from build123d import *

# Parameters (mm, degrees)
SKETCH1_W           = 50
SKETCH1_H           = 110
BOSS_EXTRUDE1_DEPTH = 10
SKETCH2_W           = 12
SKETCH2_H           = 110
BOSS_EXTRUDE2_DEPTH = 120
BOSS_EXTRUDE4_DEPTH = 152
BOSS_EXTRUDE5_DEPTH = 10
SKETCH5_W           = 152
SKETCH5_H           = 8
BOSS_EXTRUDE6_DEPTH = 10
SKETCH6_W           = 152
SKETCH6_H           = 8
BOSS_EXTRUDE7_DEPTH = 10
SKETCH7_R           = 2.5
CUT_EXTRUDE1_DEPTH  = 87
SKETCH8_W           = 26
SKETCH8_H           = 63.5
CUT_EXTRUDE2_DEPTH  = 5


with BuildPart() as part:
    # Sketch1 → Boss-Extrude1 (new body)
    with BuildSketch(Plane.XY):
        with Locations((-25, 55)):
            Rectangle(SKETCH1_W, SKETCH1_H)
    extrude(amount=BOSS_EXTRUDE1_DEPTH)

    # Sketch2 → Boss-Extrude2 (add)
    with BuildSketch(Plane(origin=(0, 0, 0), x_dir=(-1, 0, 0), z_dir=(0, 0, -1))):
        with Locations((6, 55)):
            Rectangle(SKETCH2_W, SKETCH2_H)
    extrude(amount=BOSS_EXTRUDE2_DEPTH)

    # Sketch3 → Boss-Extrude4 (add)
    with BuildSketch(Plane.ZY.offset(12)):
        Polygon((-120, 86.75), (-120, 76.75), (-114, 76.75), (-114, 33.25), (-120, 33.25), (-120, 23.25), (-104, 23.25), (-104, 86.75), align=None)
    extrude(amount=BOSS_EXTRUDE4_DEPTH)

    # Sketch4 → Boss-Extrude5 (add)
    with BuildSketch(Plane(origin=(0, 0, -120), x_dir=(-1, 0, 0), z_dir=(0, 0, -1))):
        Polygon((12, 86.75), (0, 86.75), (0, 23.25), (12, 23.25), (164, 23.25), (164, 33.25), (12, 33.25), (12, 76.75), (164, 76.75), (164, 86.75), align=None)
    extrude(amount=BOSS_EXTRUDE5_DEPTH)

    # Sketch5 → Boss-Extrude6 (add)
    with BuildSketch(Plane.XZ.offset(-76.75)):
        with Locations((-88, -126)):
            Rectangle(SKETCH5_W, SKETCH5_H)
    extrude(amount=BOSS_EXTRUDE6_DEPTH)

    # Sketch6 → Boss-Extrude7 (add)
    with BuildSketch(Plane(origin=(0, 33.25, 0), x_dir=(1, 0, 0), z_dir=(0, 1, 0))):
        with Locations((-88, 126)):
            Rectangle(SKETCH6_W, SKETCH6_H)
    extrude(amount=BOSS_EXTRUDE7_DEPTH)

    # Sketch7 → Cut-Extrude1 (cut)
    with BuildSketch(Plane.XY.offset(-104)):
        with Locations((-124, 61.25)):
            Circle(SKETCH7_R)
        with Locations((-124, 47.25)):
            Circle(SKETCH7_R)
    extrude(amount=-CUT_EXTRUDE1_DEPTH, mode=Mode.SUBTRACT)

    # Sketch8 → Cut-Extrude2 (cut)
    with BuildSketch(Plane.ZY.offset(164)):
        with Locations((-117, 55)):
            Rectangle(SKETCH8_W, SKETCH8_H)
    extrude(amount=-CUT_EXTRUDE2_DEPTH, mode=Mode.SUBTRACT)


solid = part.part
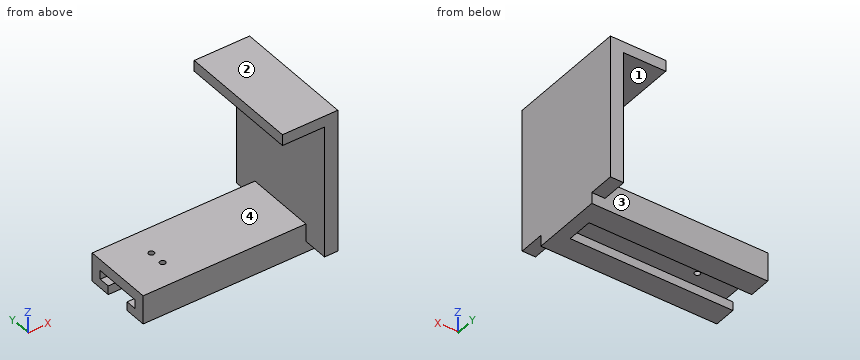
Check sheet for the modelled part. Datum: model origin and axes. Units: mm. Face numbers are marked on the shaded views. Coordinates: 2 decimals unless noted, no trailing zeros. Loops run counter-clockwise (first coordinate to the right, second up) from the corner with the lowest first, then second, coordinate; pieces in that order, holes last. Notation, with made-up numbers: (3.25, 41.5) -> (10.25, 41.5) arc R8 cw to (10.25, 50.5) -> close; hole circle Ø11 at (-9.75, 77.25). An arc over 180 degrees is marked (long way). Write item = value, one per line. Start each with the question number.
1. Draft check along Z on the marked faces 1, 2, 3 and 4. Enter one of: released by +Z, released by -Z, zero draft, split by the parting line, or undercut.
2. Depth check by flat-ended pin: P1, Ø10, axis at x = -92, z = -110, coming from the +Y side; P2, Ø17.5, axis at y = 65, z = -120, coming from the -X side; P3, Ø8, axis at x = -60.5, y = 73, coming from the +Z side; P4, Ø1.5, axis at x = -44.5, y = 96.5, coming from the -Z side. Enter the tip coordinate at first touch or a pass-through.
3. Section check C-C on x = -124. Record the cut outline in (y, z).
4. Section check A-A on y = 61.25. Record the cut outline in (x, z).
5. Material ranges on line 1 (Y direction, x = -124, z = -111); line 2 (Z direction, x = -34, y = 34); line 3 (Z direction, x = -115, y = 33.5), recorded low to high.
6. Section check D-D on y = 82. Record the cut outline in (x, z).
7. Section check B-B on x = -38. Record the cut outline in (y, z).
Responses:
q1.face_1 = undercut
q1.face_2 = released by +Z
q1.face_3 = zero draft
q1.face_4 = undercut
q2.P1 = 86.75
q2.P2 = -159
q2.P3 = -104
q2.P4 = 0
q3.outline = (23.25, -130) -> (43.25, -130) -> (43.25, -122) -> (33.25, -122) -> (33.25, -114) -> (44.75, -114) -> (44.75, -104) -> (23.25, -104) -> close; (49.75, -114) -> (58.75, -114) -> (58.75, -104) -> (49.75, -104) -> close; (63.75, -114) -> (76.75, -114) -> (76.75, -122) -> (66.75, -122) -> (66.75, -130) -> (86.75, -130) -> (86.75, -104) -> (63.75, -104) -> close
q4.outline = (-159, -114) -> (-126.5, -114) -> (-126.5, -104) -> (-159, -104) -> close; (-121.5, -114) -> (-12, -114) -> (-12, -130) -> (0, -130) -> (0, 10) -> (-50, 10) -> (-50, 0) -> (-12, 0) -> (-12, -104) -> (-121.5, -104) -> close
q5.line_1 = 23.25 to 44.75, 49.75 to 58.75, 63.75 to 86.75
q5.line_2 = -130 to -122, -114 to -104, 0 to 10
q5.line_3 = -130 to -122, -114 to -104
q6.outline = (-159, -130) -> (0, -130) -> (0, 10) -> (-50, 10) -> (-50, 0) -> (-12, 0) -> (-12, -104) -> (-159, -104) -> close
q7.outline = (0, 0) -> (110, 0) -> (110, 10) -> (0, 10) -> close; (23.25, -130) -> (43.25, -130) -> (43.25, -122) -> (33.25, -122) -> (33.25, -114) -> (76.75, -114) -> (76.75, -122) -> (66.75, -122) -> (66.75, -130) -> (86.75, -130) -> (86.75, -104) -> (23.25, -104) -> close
